Geometry: final body of the model. Coordinates: model frame, mm. Face numbers are marked on the shaded views. A direction names the side the tool comes from. Give positions to 0.01 mm unless a question says otherwise; leave off trailing zeros. Order: outer loops, then holes, each group sorted by start corner. A loop starts at its lowest first (then second) coordinate and runs counter-clockwise, first axis right, second up. Notation, with made-up numbers: (29, -32) - (54, -32) arc R26 ccw to (54, -2) - close; hole circle Ø7 at (0, -13.75). An arc over 180 degrees is marked (long way). Use one line per item in the form item = value.
from build123d import *

# Parameters (mm, degrees)
BOSS_EXTRUDE1_DEPTH             = 8
BOSS_EXTRUDE1_DEPTH_BACK        = 8
M1_6_CLEARANCE_HOLE1_AT_2_COUNT = 2
M1_6_CLEARANCE_HOLE1_AT_2_PITCH = 8.485281374
M1_6_CLEARANCE_HOLE1_AT_3_COUNT = 2
M1_6_CLEARANCE_HOLE1_AT_3_PITCH = 12
M1_6_CLEARANCE_HOLE1_AT_4_COUNT = 2
M1_6_CLEARANCE_HOLE1_AT_4_PITCH = 8.485281374
CUT_EXTRUDE1_DEPTH              = 43.093229859
CUT_EXTRUDE1_DEPTH_BACK         = 43.093229859
CUT_EXTRUDE2_DEPTH              = 43.093229859
CUT_EXTRUDE2_DEPTH_BACK         = 43.093229859
SKETCH6_W                       = 6
SKETCH6_H                       = 1.8
SKETCH6_W_2                     = 12
SKETCH6_H_2                     = 4.4
BOSS_EXTRUDE2_START             = -0.5
SKETCH8_W                       = 23
SKETCH8_H                       = 7
BOSS_EXTRUDE2_DEPTH             = 1.6
BOSS_EXTRUDE3_DEPTH             = 7
BOSS_EXTRUDE4_DEPTH             = 1.55
SKETCH13_W                      = 16
SKETCH13_H                      = 6.4
BOSS_EXTRUDE5_DEPTH             = 1
BOSS_EXTRUDE6_DEPTH             = 1.5
BOSS_EXTRUDE6_DEPTH_BACK        = 1.5
FILLET1_R                       = 0.6
FILLET2_R                       = 10
FILLET3_R                       = 3
CUT_EXTRUDE3_DEPTH              = 66.244463379
CUT_EXTRUDE3_DEPTH_BACK         = 10
SKETCH16_R                      = 3


with BuildPart() as part:
    # Sketch1 → Boss-Extrude1 (new, two sides: drawn at the far end of the back side and taken through both)
    with BuildSketch(Plane.XY.offset(-BOSS_EXTRUDE1_DEPTH_BACK)):
        Polygon((18.6, 18), (-18.6, 18), (-18.6, -18), (-14.6, -18), (-14.6, 10), (14.6, 10), (14.6, -18), (18.6, -18), align=None)
    extrude(amount=BOSS_EXTRUDE1_DEPTH + BOSS_EXTRUDE1_DEPTH_BACK)

    # Sketch4 → M1.6 Clearance Hole1 (revolve, cut)
    with BuildSketch(Plane(origin=(18.6, -3.8, 6), x_dir=(0, 0, -1), z_dir=(0, 1, 0))):
        Polygon((0, 0), (0, 4.600860619), (1, 4), (1, 0.025), (1.025, 0), align=None)
    m1_6_clearance_hole1 = revolve(axis=Axis((24.95, -3.8, 6), (-1, 0, 0)), mode=Mode.SUBTRACT)

    # M1.6 Clearance Hole1 at 2: M1.6 Clearance Hole1 ×2
    with Locations(*[Vector(0, 0.7071067811865476, -0.7071067811865476) * (i * M1_6_CLEARANCE_HOLE1_AT_2_PITCH) for i in range(1, M1_6_CLEARANCE_HOLE1_AT_2_COUNT)]):
        add(m1_6_clearance_hole1, mode=Mode.SUBTRACT)

    # M1.6 Clearance Hole1 at 3: M1.6 Clearance Hole1 ×2
    with Locations(*[(0, 0, -i * M1_6_CLEARANCE_HOLE1_AT_3_PITCH) for i in range(1, M1_6_CLEARANCE_HOLE1_AT_3_COUNT)]):
        add(m1_6_clearance_hole1, mode=Mode.SUBTRACT)

    # M1.6 Clearance Hole1 at 4: M1.6 Clearance Hole1 ×2
    with Locations(*[Vector(0, -0.7071067811865475, -0.7071067811865476) * (i * M1_6_CLEARANCE_HOLE1_AT_4_PITCH) for i in range(1, M1_6_CLEARANCE_HOLE1_AT_4_COUNT)]):
        add(m1_6_clearance_hole1, mode=Mode.SUBTRACT)

    # Mirror1: M1.6 Clearance Hole1 across plane
    add(m1_6_clearance_hole1.mirror(Plane(origin=(0, 0, 0), x_dir=(0, 0, 1), z_dir=(1, 0, 0))), mode=Mode.SUBTRACT)

    # Mirror1 copy 1 sketch → Mirror1 copy 1 (revolve, cut)
    with BuildSketch(Plane(origin=(-18.6, 2.2, 0), x_dir=(0, 0, -1), z_dir=(0, 1, 0))):
        Polygon((0, 0), (0, -4.600860619), (1, -4), (1, -0.025), (1.025, 0), align=None)
    revolve(axis=Axis((-24.95, 2.2, 0), (-1, 0, 0)), mode=Mode.SUBTRACT)

    # Mirror1 copy 2 sketch → Mirror1 copy 2 (revolve, cut)
    with BuildSketch(Plane(origin=(-18.6, -3.8, -6), x_dir=(0, 0, -1), z_dir=(0, 1, 0))):
        Polygon((0, 0), (0, -4.600860619), (1, -4), (1, -0.025), (1.025, 0), align=None)
    revolve(axis=Axis((-24.95, -3.8, -6), (-1, 0, 0)), mode=Mode.SUBTRACT)

    # Mirror1 copy 3 sketch → Mirror1 copy 3 (revolve, cut)
    with BuildSketch(Plane(origin=(-18.6, -9.8, 0), x_dir=(0, 0, -1), z_dir=(0, 1, 0))):
        Polygon((0, 0), (0, -4.600860619), (1, -4), (1, -0.025), (1.025, 0), align=None)
    revolve(axis=Axis((-24.95, -9.8, 0), (-1, 0, 0)), mode=Mode.SUBTRACT)

    # Sketch5 → Cut-Extrude1 (cut, two sides: drawn at the far end of the back side and taken through both)
    with BuildSketch(Plane(origin=(18.6, 0, 0), x_dir=(0, 0, -1), z_dir=(1, 0, 0)).offset(-CUT_EXTRUDE1_DEPTH_BACK)):
        with BuildLine():
            Line((-8, -3.8), (-8, -18))
            Line((-8, -18), (8, -18))
            Line((8, -18), (8, -3.8))
            ThreePointArc((8, -3.8), (0, -11.8), (-8, -3.8))
        make_face()
    extrude(amount=CUT_EXTRUDE1_DEPTH + CUT_EXTRUDE1_DEPTH_BACK, mode=Mode.SUBTRACT)

    # Sketch6 → Cut-Extrude2 (cut, two sides: drawn at the far end of the back side and taken through both)
    with BuildSketch(Plane.ZY.offset(18.6).offset(-CUT_EXTRUDE2_DEPTH_BACK)):
        with Locations((0, 17.1)):
            Rectangle(SKETCH6_W, SKETCH6_H)
        with Locations((0, 14)):
            Rectangle(SKETCH6_W_2, SKETCH6_H_2)
    extrude(amount=CUT_EXTRUDE2_DEPTH + CUT_EXTRUDE2_DEPTH_BACK, mode=Mode.SUBTRACT)

    # Sketch8 → Boss-Extrude2 (add)
    with BuildSketch(Plane(origin=(0, 11.8, 0), x_dir=(1, 0, 0), z_dir=(0, 1, 0)).offset(BOSS_EXTRUDE2_START)):
        with Locations((-30.1, 0)):
            Rectangle(SKETCH8_W, SKETCH8_H)
    extrude(amount=-BOSS_EXTRUDE2_DEPTH)

    # Sketch10 → Boss-Extrude3 (add)
    with BuildSketch(Plane.XY.offset(3.5)):
        Polygon((-41.6, 11.3), (-43.6, 11.3), (-43.6, 2.3), (-37.6, 2.3), (-37.6, 4.3), (-41.6, 4.3), align=None)
    extrude(amount=-BOSS_EXTRUDE3_DEPTH)

    # Sketch12 → Boss-Extrude4 (add)
    with BuildSketch(Plane(origin=(18.6, 0, 0), x_dir=(0, 0, -1), z_dir=(1, 0, 0))):
        Polygon((6, 11.8), (6, 16.2), (8, 16.2), (8, 9.8), (-8, 9.8), (-8, 16.2), (-6, 16.2), (-6, 11.8), align=None)
    extrude(amount=BOSS_EXTRUDE4_DEPTH)

    # Sketch13 → Boss-Extrude5 (add)
    with BuildSketch(Plane(origin=(20.15, 0, 0), x_dir=(0, 0, -1), z_dir=(1, 0, 0))):
        with Locations((0, 13)):
            Rectangle(SKETCH13_W, SKETCH13_H)
    extrude(amount=BOSS_EXTRUDE5_DEPTH)

    # Sketch14 → Boss-Extrude6 (add, two sides: drawn at the far end of the back side and taken through both)
    with BuildSketch(Plane.XY.offset(-BOSS_EXTRUDE6_DEPTH_BACK)):
        Polygon((-41.7, 11.3), (-41.7, 12.3), (-38.7, 13.5), (-38.7, 11.3), align=None)
    extrude(amount=BOSS_EXTRUDE6_DEPTH + BOSS_EXTRUDE6_DEPTH_BACK)

    # Fillet1
    fillet1_edges = [part.edges().sort_by_distance(p)[0] for p in [
        (-41.7, 12.3, 0),
    ]]
    fillet(fillet1_edges, radius=FILLET1_R)

    # Fillet2
    # the kernel refuses this fillet: 10 mm, written as the material it adds along each edge
    with BuildSketch(Plane(origin=(-18.6, 11.3, -3.5), x_dir=(-1.5292458657399207e-12, 0, -1.0), z_dir=(0, -1, 0))) as fillet2_piece_1:
        with BuildLine():
            CenterArc((10, -8.351646544), FILLET2_R, 123.367012969, 56.632987031)
            Line((0, -8.351646544), (0, 0))
            Line((0, 0), (4.5, 0))
        make_face()
    extrude(amount=1.6)
    with BuildSketch(Plane(origin=(-18.6, 11.3, 3.5), x_dir=(-1, 0, 0), z_dir=(0, -1, 0))) as fillet2_piece_2:
        with BuildLine():
            CenterArc((8.351646544, -10), FILLET2_R, 90, 56.632987031)
            Line((0, -4.5), (0, 0))
            Line((0, 0), (8.351646544, 0))
        make_face()
    extrude(amount=1.6)

    # Fillet3
    # the kernel refuses this fillet: 3 mm, written as the material it adds along each edge
    with BuildSketch(Plane(origin=(-18.6, 9.7, 3.5), x_dir=(-1, 0, 0), z_dir=(0, 0, -1))) as fillet3_piece_1:
        with BuildLine():
            CenterArc((FILLET3_R, -FILLET3_R), FILLET3_R, 90, 90)
            Line((0, -FILLET3_R), (0, 0))
            Line((0, 0), (FILLET3_R, 0))
        make_face()
    extrude(amount=7)
    with BuildSketch(Plane(origin=(-18.6, 9.7, 8), x_dir=(-1.0, 0, -1.5555555555538275e-12), z_dir=(1.5555555555538273e-12, 0, -1.0))) as fillet3_piece_2_section:
        with BuildLine():
            CenterArc((FILLET3_R, -FILLET3_R), FILLET3_R, 90, 90)
            Line((0, -FILLET3_R), (0, 0))
            Line((0, 0), (FILLET3_R, 0))
        make_face()
    fillet3_piece_2 = extrude(amount=4.5, mode=Mode.PRIVATE)
    fillet3_piece_2 = fillet3_piece_2 - Plane(origin=(-26.951646544, 8.943750406, 13.5), x_dir=(-1, 0, 0), z_dir=(0, 1, 0)) * Cylinder(10, 22, mode=Mode.PRIVATE)
    add(fillet3_piece_2)
    with BuildSketch(Plane(origin=(-18.6, 9.7, -3.5), x_dir=(-1.0, 0, 2e-12), z_dir=(-2e-12, 0, -1.0))) as fillet3_piece_3_section:
        with BuildLine():
            CenterArc((FILLET3_R, -FILLET3_R), FILLET3_R, 90, 90)
            Line((0, -FILLET3_R), (0, 0))
            Line((0, 0), (FILLET3_R, 0))
        make_face()
    fillet3_piece_3 = extrude(amount=4.5, mode=Mode.PRIVATE)
    fillet3_piece_3 = fillet3_piece_3 - Plane(origin=(-26.951646544, 8.943748833, -13.5), x_dir=(-2e-12, 0, -1.0), z_dir=(0, 1, 0)) * Cylinder(10, 22, mode=Mode.PRIVATE)
    add(fillet3_piece_3)

    # Sketch16 → Cut-Extrude3 (cut, two sides: drawn at the far end of the back side and taken through both)
    with BuildSketch(Plane(origin=(18.6, 0, 0), x_dir=(0, 0, -1), z_dir=(1, 0, 0)).offset(-CUT_EXTRUDE3_DEPTH_BACK)):
        with Locations(Location((0, -3.8, 0), (0, 0, 180))):
            Circle(SKETCH16_R)
    extrude(amount=CUT_EXTRUDE3_DEPTH + CUT_EXTRUDE3_DEPTH_BACK, mode=Mode.SUBTRACT)


solid = part.part
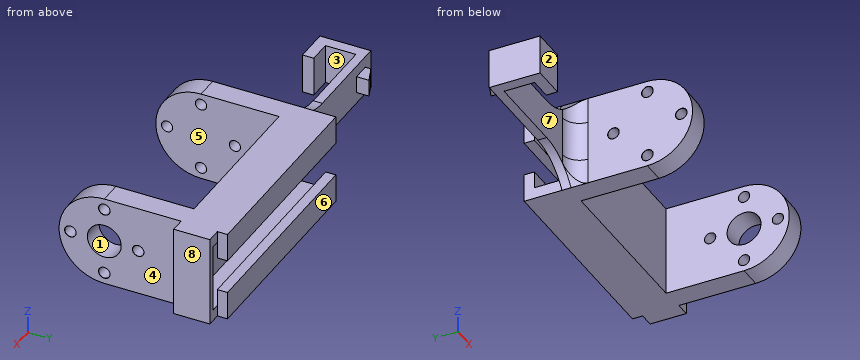
(1) Cut plane A-A on y = 6. Output: boundary loops of the cut face in (x, z).
Computed values:
outline = (-43.6, -3.5) - (-41.6, -3.5) - (-41.6, 3.5) - (-43.6, 3.5) - close; (-18.6, -8) - (-14.6, -8) - (-14.6, 8) - (-18.6, 8) - close; (14.6, -8) - (18.6, -8) - (18.6, 8) - (14.6, 8) - close
(2) Reachability of the marked faces 1, 2, 3, 4 and 5 from +Z, -Z, +X, -X, +Y, -Y: full face, straight path, thin tool, end or side. Return the list, or none.
Computed values:
face_1 = +X
face_2 = +Z, -Z, -X, -Y
face_3 = +Z, -Z
face_4 = +Z, -Z, +X, -Y
face_5 = +Z, -Z, -Y
(3) Pull-direction query (Y, two-part tool) for the marked faces 6, 7 and 8; classes: released by +Y, released by -Y, zero draft, split by the parting line, or undercut.
Computed values:
face_6 = released by +Y
face_7 = undercut
face_8 = zero draft
(4) Cut plane B-B on z = -2.25. Output: boundary loops of the cut face in (x, y), plus the area to 3 significant figures.
Computed values:
outline = (-43.6, 2.3) - (-37.6, 2.3) - (-37.6, 4.3) - (-41.6, 4.3) - (-41.6, 9.7) - (-21.6, 9.7) arc R3 cw to (-18.6, 6.7) - (-18.6, -11.48) - (-14.6, -11.48) - (-14.6, 10) - (14.6, 10) - (14.6, -1.82) - (18.6, -1.82) - (18.6, 9.8) - (21.15, 9.8) - (21.15, 16.2) - (20.15, 16.2) - (20.15, 11.8) - (-18.6, 11.8) - (-18.6, 11.3) - (-43.6, 11.3) - close; (14.6, -11.48) - (18.6, -11.48) - (18.6, -5.78) - (14.6, -5.78) - close
area = 297 mm²
(5) Cut plane C-C on y = -9.8. Give the number of separate pieces and of enclosed holes in the cut face, plus the area to 3 significant figures.
Computed values:
separate_pieces = 4
enclosed_holes = 0
area = 68.7 mm²
(6) Ray query, line 1 along X through (y, z) = (4.5, 1.5); line 2 along Z through (x, y) = (-2, 13); line 3 along Y through (x, z) = (-39.5, 3.25). Return the intervals inside material, ascending.
Computed values:
line_1 = -43.6 to -41.6, -18.6 to -14.6, 14.6 to 18.6
line_2 = -8 to -6, 6 to 8
line_3 = 2.3 to 4.3, 9.7 to 11.3
(7) Contact query for flat-ended pins moving along their axis: pin 1 Ø2.5 at (y, z) = (-3.8, 6) entering from +X; pin 2 Ø8 at (y, z) = (-3, -5.5) entering from -X; pin 3 Ø3 at (x, z) = (-27.5, 6) entering from +Y; pin 4 Ø1.8 at (x, z) = (-41.5, -1.5) entering from -Y. Output: stop coordinate, or through.
Computed values:
pin_1 = 18.6
pin_2 = -18.6
pin_3 = through
pin_4 = 2.3
(8) Cut plane D-D on x = -14. Output: boundary loops of the cut face in (y, z), plus the area to 3 significant figures.
Computed values:
outline = (10, -8) - (18, -8) - (18, -3) - (16.2, -3) - (16.2, -6) - (11.8, -6) - (11.8, 6) - (16.2, 6) - (16.2, 3) - (18, 3) - (18, 8) - (10, 8) - close
area = 64.4 mm²
